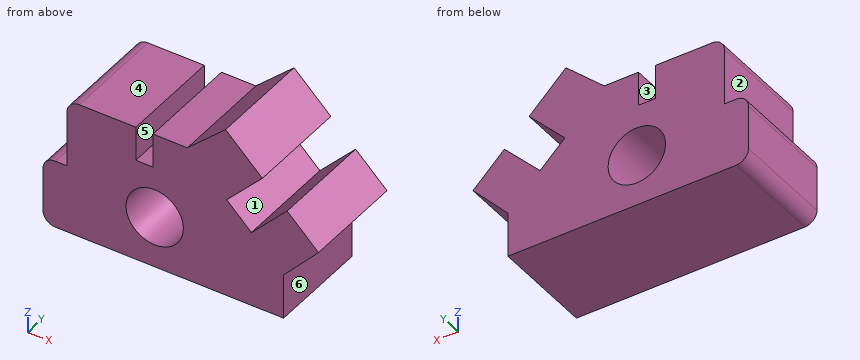
```python
from build123d import *

# Parameters (mm, degrees)
F0_R     = 8.350726
F1_DEPTH = 30


with BuildPart() as f1:
    # F0 (on Front) → F1 (new body)
    with BuildSketch(Plane.XZ):
        with BuildLine():
            Line((-54.655215, -25.540138), (11.771582, -25.540138))
            Line((11.771582, -25.540138), (11.771582, -12.473472))
            Line((11.771582, -12.473472), (21.932656, -1.439317))
            Line((21.932656, -1.439317), (12.803844, 7.34173))
            Line((12.803844, 7.34173), (2.407616, -3.466229))
            Line((2.407616, -3.466229), (-4.799395, 3.466229))
            Line((-4.799395, 3.466229), (5.599293, 14.276747))
            Line((5.599293, 14.276747), (-5.112314, 24.580292))
            Line((-5.112314, 24.580292), (-16.22842, 14.459862))
            Line((-16.22842, 14.459862), (-26.22842, 14.459862))
            Line((-26.22842, 14.459862), (-26.22842, 4.459862))
            Line((-26.22842, 4.459862), (-31.22842, 4.459862))
            Line((-31.22842, 4.459862), (-31.22842, 14.459862))
            Line((-31.22842, 14.459862), (-47.655217, 14.459862))
            ThreePointArc((-47.655217, 14.459862), (-50.181853, 13.413295), (-51.22842, 10.886659))
            Line((-51.22842, 10.886659), (-51.22842, -5.540138))
            Line((-51.22842, -5.540138), (-54.655215, -5.540138))
            ThreePointArc((-54.655215, -5.540138), (-57.181851, -6.586705), (-58.228418, -9.113341))
            Line((-58.228418, -9.113341), (-58.228418, -21.966935))
            ThreePointArc((-58.228418, -21.966935), (-57.181851, -24.493571), (-54.655215, -25.540138))
        make_face()
        with Locations((-25.728418, -10.540138)):
            Circle(F0_R, mode=Mode.SUBTRACT)
    extrude(amount=F1_DEPTH)


solid = f1.part
```
Geometry: final body of the model. Coordinates: model frame, mm. Face numbers are marked on the shaded views. A direction names the side the tool comes from. Round coordinates to 2 decimals unless told otherwise and drop trailing zeros. Loops run counter-clockwise (first coordinate to the right, second up) from the corner with the lowest first, then second, coordinate; pieces in that order, holes last. Notation, with made-up numbers: (71.5, 84) -> (76.5, 84) arc R20 cw to (76.5, 92) -> close; hole circle Ø3 at (-23.75, 85.5). An arc over 180 degrees is marked (long way). Use one line per item in the form item = value. Start each with the question number.
1) First-contact query: P1, Ø3, axis at y = -15.5, z = 9.5, coming from the +X side; P2, Ø2.5, axis at x = -28.5, y = -20, coming from the +Z side; P3, Ø3, axis at y = -18, z = 11, coming from the -X side; P4, Ø1, axis at y = -8.5, z = -1, coming from the +X side. Flat tips, straight axial feed; report the tip coordinate or a pass-through.
2) Section D-D on x = -52.5. Output: boundary loops of the cut face in (y, z), then the cut area to 3 significant figures.
3) Line query: L1, parallel to Z at x = -48, y = -28; L2, parallel to X at y = -21.25, z = -20; L3, parallel to Z at x = -38, y = -26.5. Output: solid intervals per line, ascending.
4) Section B-B on y = -16.25. Output: boundary loops of the cut face in (x, z).
5) Access query for the marked faces 1, 2 and 3. Directions: +Z, -Z, +X, -X, +Y, -Y. A direction counts if a zero-diameter tool reaches every point of the face in a straight line with its end or side. Return the directions, or none.
6) Draft query along X for the marked faces 4, 5 and 6. Return one class per face: released by +X, released by -X, zero draft, split by the parting line, or undercut.
7) Section A-A on z = -17. Output: boundary loops of the cut face in (x, y).
8) Section C-C on x = -35. Output: boundary loops of the cut face in (y, z), then the cut area to 3 significant figures.
Response:
q1.P1 = 2.45
q1.P2 = 4.46
q1.P3 = -51.23
q1.P4 = 21.93
q2.outline = (-30, -25.54) -> (0, -25.54) -> (0, -5.54) -> (-30, -5.54) -> close
q2.area = 600 mm^2
q3.L1 = -25.54 to 14.44
q3.L2 = -58.23 to 11.77
q3.L3 = -25.54 to 14.46
q4.outline = (-58.23, -21.97) arc R3.57 ccw to (-54.66, -25.54) -> (11.77, -25.54) -> (11.77, -12.47) -> (21.93, -1.44) -> (12.8, 7.34) -> (2.41, -3.47) -> (-4.8, 3.47) -> (5.6, 14.28) -> (-5.11, 24.58) -> (-16.23, 14.46) -> (-26.23, 14.46) -> (-26.23, 4.46) -> (-31.23, 4.46) -> (-31.23, 14.46) -> (-47.66, 14.46) arc R3.57 ccw to (-51.23, 10.89) -> (-51.23, -5.54) -> (-54.66, -5.54) arc R3.57 ccw to (-58.23, -9.11) -> close; hole circle Ø16.7 at (-25.73, -10.54)
q5.face_1 = +Y, -Y
q5.face_2 = +Z, -X, +Y, -Y
q5.face_3 = +Z, +Y, -Y
q6.face_4 = zero draft
q6.face_5 = undercut
q6.face_6 = released by +X
q7.outline = (-58.23, -30) -> (-31.02, -30) -> (-31.02, 0) -> (-58.23, 0) -> close; (-20.44, -30) -> (11.77, -30) -> (11.77, 0) -> (-20.44, 0) -> close
q8.outline = (-30, -25.54) -> (0, -25.54) -> (0, 14.46) -> (-30, 14.46) -> close
q8.area = 1,200 mm^2
